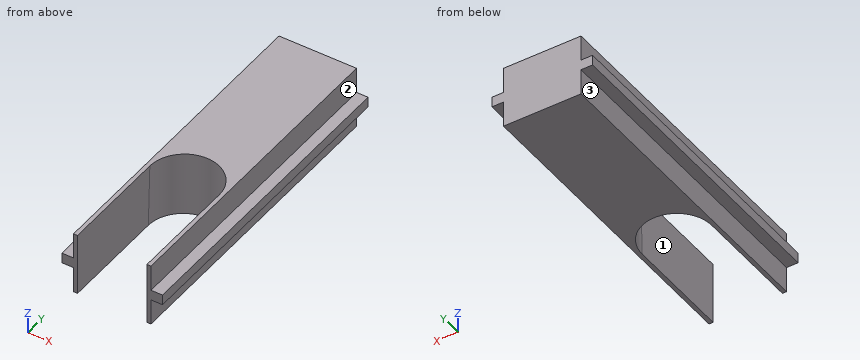
Autodesk Inventor part; units mm, degrees
ref_plane "YZ Plane" through (0, 0, 0) normal (1, 0, 0) x (0, 1, 0)
ref_plane "XZ Plane" through (0, 0, 0) normal (0, 1, 0) x (-1, 0, 0)
ref_plane "XY Plane" through (0, 0, 0) normal (0, 0, 1) x (1, 0, 0)
sketch "草圖1" plane through (0, 0, 0) normal (0, 1, 0) x (-1, 0, 0)
  line L0 (-33.5, 27) -> (33.5, 27)
  line L1 (33.5, 27) -> (33.5, -27)
  line L2 (33.5, -27) -> (-33.5, -27)
  line L3 (-33.5, -27) -> (-33.5, 27)
  line L4 (-33.5, 27) -> (33.5, -27) construction
  line L5 (33.5, 27) -> (-33.5, -27) construction
  line L6 (43.5, -4.5) -> (33.5, -4.5)
  line L7 (33.5, -4.5) -> (33.5, 4.5)
  line L8 (33.5, 4.5) -> (43.5, 4.5)
  line L9 (43.5, 4.5) -> (43.5, -4.5)
  line L10 (-33.5, -4.5) -> (-43.5, -4.5)
  line L11 (-43.5, -4.5) -> (-43.5, 4.5)
  line L12 (-43.5, 4.5) -> (-33.5, 4.5)
  line L13 (-33.5, 4.5) -> (-33.5, -4.5)
  point P0 (0, 0)
  point P1 (33.5, 0)
  point P2 (-33.5, 0)
  point P3 (-33.5, 4.5)
  point P4 (-33.5, -4.5)
  dimension "d0" = 67
  dimension "d1" = 54
  dimension "d2" = 9
  dimension "d3" = 10
extrude "擠出1" add sketch "草圖1" along normal blind 400
sketch "草圖2" plane through (-33.5, 0, 27) normal (0, 0, 1) x (1, 0, 0)
  line L0 (0, 0) -> (0, 400)
  line L1 (0, 400) -> (67, 400)
  line L2 (67, 400) -> (67, 0)
  line L3 (67, 0) -> (0, 0)
  circle A0 centre (33.5, 199) radius 30
  line L4 (3.5, 199) -> (63.5, 199)
  line L5 (63.5, 199) -> (63.5, -2.327)
  line L6 (63.5, -2.327) -> (3.5, -2.327)
  line L7 (3.5, -2.327) -> (3.5, 199)
  point P0 (33.5, 0)
  point P1 (33.5, 0)
  point P2 (3.5, 199)
  point P3 (3.5, 0)
  point P4 (63.5, 0)
  dimension "d6" = 199
  dimension "d7" = 60
extrude "擠出2" cut sketch "草圖2" against normal through all contours L7 A0 L5 L3 | L4 A0 | A0 L4
sketch "草圖3" plane through (-33.5, 400, 27) normal (0, 0, 1) x (1, 0, 0)
  line L0 (-79.9627, -270) -> (146.9627, -270)
  line L1 (146.9627, -270) -> (146.9627, -400)
  line L2 (146.9627, -400) -> (-79.9627, -400)
  line L3 (-79.9627, -400) -> (-79.9627, -270)
  point P0 (33.5, -400)
  point P1 (33.5, -400)
  dimension "d10" = 130
extrude "擠出3" cut sketch "草圖3" against normal through all
sketch "草圖4" plane through (33.5, 400, -27) normal (0, 0, -1) x (-1, 0, 0)
  arc A0 (63.5, -201) -> (3.5, -201) centre (33.5, -201) ccw construction
  circle A1 centre (33.5, -177) radius 30
  line L0 (63.5, -270) -> (3.5, -270)
  line L1 (3.5, -270) -> (3.5, -177)
  line L2 (3.5, -177) -> (63.5, -177)
  line L3 (63.5, -177) -> (63.5, -270)
  point P0 (33.5, -400)
  point P1 (63.5, -270)
  dimension "d13" = 24
  dimension "d14" = 60
sketch "草圖5" plane through (-33.5, 400, 27) normal (0, 0, 1) x (1, 0, 0)
  circle A0 centre (33.5, -175) radius 30
  arc A1 (63.5, -201) -> (3.5, -201) centre (33.5, -201) ccw
  line L0 (63.5, -270) -> (3.5, -270)
  line L1 (3.5, -270) -> (3.5, -175)
  line L2 (3.5, -175) -> (63.5, -175)
  line L3 (63.5, -175) -> (63.5, -270)
  point P0 (33.5, -400)
  point P1 (63.5, -270)
  dimension "d15" = 26
  dimension "d16" = 60
loft "斷面混成1" cut profiles "草圖4", "草圖5"
properties part number "Slider-7"
Here's how the part is built. I have some questions about the finished solid (model axes, mm). Face numbers are marked on the shaded views. A direction names the side the tool comes from. Give positions to 0.01 mm unless a question says otherwise; leave off trailing zeros. Order: outer loops, then holes, each group sorted by start corner. A loop starts at its lowest first (then second) coordinate and runs counter-clockwise, first axis right, second up. Notation, with made-up numbers: (63.25, 77) -> (106.25, 77) arc R22 cw to (106.25, 113) -> close; hole circle Ø9 at (80.25, 51.5). An arc over 180 degrees is marked (long way). Use a Markdown table: item, result. Add a question column.
Item 1: For the marked faces 1, 2 and 3, which set-ups out of +Z, -Z, +X, -X, +Y, -Y let a thin tool reach every point of the face, with its end or its side?
Item 2: I need wall thicknesses on line 1 (X direction, y = 203, z = 1.5); line 2 (X direction, y = 173.5, z = 12.5); line 3 (X direction, y = 370, z = -8). Which ranges of each line are inside material? Lowest first, please.
Item 3: Will these pins go through, and if not, where does the flat tip stop? pin 1 (7 mm diameter, centred on y = 252.5, z = -15.5, fed in from +X); pin 2 (1 mm diameter, centred on y = 314.5, z = 10, fed in from -X); pin 3 (11 mm diameter, centred on x = -39.5, y = 250.5, fed in from -Z).
Item 4: Imagine slicing it at B-B on y = 329. Please give me the cut outline in (x, z), plus the area to 3 significant figures.
Item 5: Imagine slicing it at A-A on y = 151. Please give me the cut outline in (x, z).
Data:
| question | item | result |
|---|---|---|
| 1 | face 1 | +Z, -Z, -Y |
| 1 | face 2 | +Z, +X, +Y, -Y |
| 1 | face 3 | -Z, -X, +Y, -Y |
| 2 | line 1 | x = -43.5 to -30, 30 to 43.5 |
| 2 | line 2 | x = -33.5 to -30, 30 to 33.5 |
| 2 | line 3 | x = -33.5 to 33.5 |
| 3 | pin 1 | stops at x = 33.5 |
| 3 | pin 2 | stops at x = -33.5 |
| 3 | pin 3 | stops at z = -4.5 |
| 4 | outline | (-43.5, -4.5) -> (-33.5, -4.5) -> (-33.5, -27) -> (33.5, -27) -> (33.5, -4.5) -> (43.5, -4.5) -> (43.5, 4.5) -> (33.5, 4.5) -> (33.5, 27) -> (-33.5, 27) -> (-33.5, 4.5) -> (-43.5, 4.5) -> close |
| 4 | area | 3,800 mm² |
| 5 | outline | (-43.5, -4.5) -> (-33.5, -4.5) -> (-33.5, -27) -> (-30, -27) -> (-30, 27) -> (-33.5, 27) -> (-33.5, 4.5) -> (-43.5, 4.5) -> close; (30, -27) -> (33.5, -27) -> (33.5, -4.5) -> (43.5, -4.5) -> (43.5, 4.5) -> (33.5, 4.5) -> (33.5, 27) -> (30, 27) -> close |
